The listing builds one solid part. Answer for the finished solid, in the listing's coordinates (mm). Face numbers are marked on the shaded views. A direction names the side the tool comes from. Round coordinates to 2 decimals unless told otherwise and drop trailing zeros. Write each loop counter-clockwise with the first axis right and the second up, starting at its lowest first coordinate (ties: lowest second). Pieces come first, ordered by that corner, then holes.
Item 1: For a pull along Z with two mould halves and no side action, classify the marked faces 4, 5 and 6 as +Z half, -Z half, draft (parallel to the pull), parting line (faces both ways), or undercut.
Item 2: Find section B-B on z = 10.25. Give the vertices of the cut face in (x, y).
Item 3: Each of these flat-tipped pins is pushed along its axis until it touches: pin 1 (4 mm diameter, centred on y = -17, z = 6.5, fed in from -X); pin 2 (2.5 mm diameter, centred on y = 20, z = 8, fed in from +X). Where does it stop, or does it pass through?
Item 4: Find section C-C on x = 0. Give the vertices of the cut face in (y, z), then the cut area to 3 significant figures.
Item 5: Find section D-D on y = 20. Give the vertices of the cut face in (x, z).
Item 6: Find the intervals of material crossed by probe 1 along Y at (x, z) = (-1, 11.25); probe 2 along Z at (x, y) = (0, -26.5); probe 3 along X at (y, z) = (24.5, 6), in increasing order.
Item 7: A tool of negligible diameter and unlimited length cuts with its end or side. For the marked faces 1, 2 and 3, from which of +Z, -Z, +X, -X, +Y, -Y can it reach the whole face along a straight path? Write none if from no direction.
Item 8: Find section A-A on z = 6. Give the vertices of the cut face in (x, y).
```python
from build123d import *

# Parameters (mm, degrees)
DODANIE_WYCI_GNI_CIE1_DEPTH = 12
WYTNIJ_WYCI_GNI_CIE1_START  = 32
SZKIC2_R                    = 3
WYTNIJ_WYCI_GNI_CIE1_DEPTH  = 12
WYTNIJ_WYCI_GNI_CIE2_START  = -20
SZKIC2_2_R                  = 3
WYTNIJ_WYCI_GNI_CIE2_DEPTH  = 12


with BuildPart() as part:
    # Szkic1 → Dodanie-wyciągnięcie1 (new body)
    with BuildSketch(Plane.XY):
        Polygon((-25.5, -22), (-25.5, -32), (25.5, -32), (25.5, 14), (-17.5, 14), (-17.5, 22), (25.5, 22), (25.5, 32), (-25.5, 32), (-25.5, -14), (17.5, -14), (17.5, -21.960784314), align=None)
    extrude(amount=DODANIE_WYCI_GNI_CIE1_DEPTH)

    # Szkic2 → Wytnij-wyciągnięcie1 (cut)
    with BuildSketch(Plane(origin=(0, 0, 0), x_dir=(1, 0, 0), z_dir=(0, 1, 0)).offset(WYTNIJ_WYCI_GNI_CIE1_START)):
        with Locations(Location((0, -6, 0), (0, 0, 270))):
            Circle(SZKIC2_R)
    extrude(amount=-WYTNIJ_WYCI_GNI_CIE1_DEPTH, mode=Mode.SUBTRACT)

    # Szkic2<2> → Wytnij-wyciągnięcie2 (cut)
    with BuildSketch(Plane(origin=(0, 0, 0), x_dir=(1, 0, 0), z_dir=(0, 1, 0)).offset(WYTNIJ_WYCI_GNI_CIE2_START)):
        with Locations(Location((0, -6, 0), (0, 0, 270))):
            Circle(SZKIC2_2_R)
    extrude(amount=-WYTNIJ_WYCI_GNI_CIE2_DEPTH, mode=Mode.SUBTRACT)


solid = part.part
```
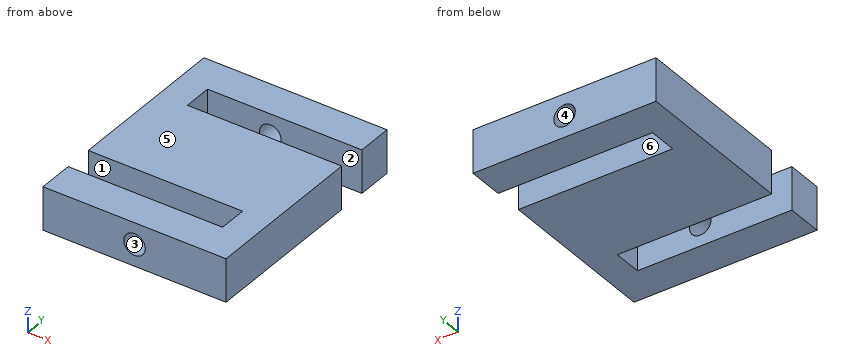
Check values:
1. face 4: undercut
1. face 5: +Z half
1. face 6: draft
2. outline: (-25.5, -32) - (25.5, -32) - (25.5, 14) - (-17.5, 14) - (-17.5, 22) - (25.5, 22) - (25.5, 32) - (-25.5, 32) - (-25.5, -14) - (17.5, -14) - (17.5, -21.96) - (-25.5, -22) - close
3. pin 1: stops at x = 17.5
3. pin 2: stops at x = -17.5
4. outline: (-32, 0) - (-21.98, 0) - (-21.98, 3) - (-32, 3) - close; (-32, 9) - (-21.98, 9) - (-21.98, 12) - (-32, 12) - close; (-14, 0) - (14, 0) - (14, 12) - (-14, 12) - close; (22, 0) - (32, 0) - (32, 3) - (22, 3) - close; (22, 9) - (32, 9) - (32, 12) - (22, 12) - close
4. area: 456 mm2
5. outline: (-25.5, 0) - (-17.5, 0) - (-17.5, 12) - (-25.5, 12) - close
6. probe 1: y = -32 to -21.98, -14 to 14, 22 to 32
6. probe 2: z = 0 to 3, 9 to 12
6. probe 3: x = -25.5 to -3, 3 to 25.5
7. face 1: +Z, -Z, -X
7. face 2: +Z, -Z, +X
7. face 3: -Y
8. outline: (-25.5, -32) - (-3, -32) - (-3, -21.98) - (-25.5, -22) - close; (-25.5, -14) - (17.5, -14) - (17.5, -21.96) - (3, -21.97) - (3, -32) - (25.5, -32) - (25.5, 14) - (-17.5, 14) - (-17.5, 22) - (-3, 22) - (-3, 32) - (-25.5, 32) - close; (3, 22) - (25.5, 22) - (25.5, 32) - (3, 32) - close
